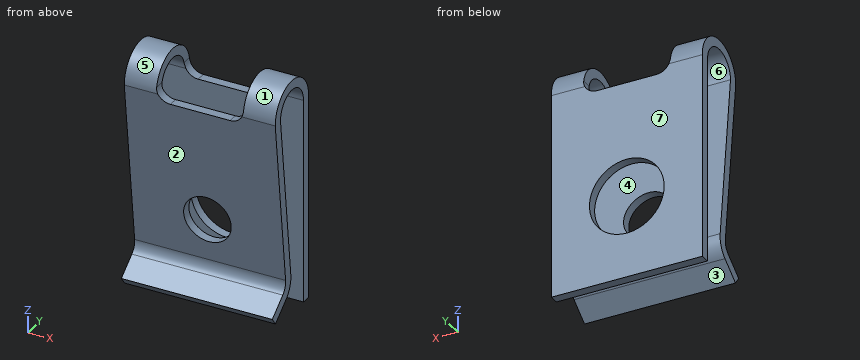
from build123d import *

# Parameters (mm, degrees)
F1_DEPTH = 5.56
F2_W     = 6.4
F2_H     = 3.95
F2_H_2   = 0.55
F2_R     = 1.75
F3_DEPTH = 4.901
F2_R_2   = 2.75
F4_DEPTH = 0.7
F5_R     = 1
F6_R     = 1.7


with BuildPart() as f1:
    # F0 (on Right) → F1 (new body, symmetric)
    with BuildSketch(Plane.YZ):
        with BuildLine():
            Line((1.55, -15), (2.25, -15))
            Line((2.25, -15), (2.25, 0))
            ThreePointArc((2.25, 0), (0, 2.25), (-2.25, 0))
            Line((-2.25, 0), (-0.790171, -12.749847))
            Line((-0.790171, -12.749847), (-2.65, -14.197634))
            Line((-2.65, -14.197634), (-2.22001, -14.75))
            Line((-2.22001, -14.75), (-0.05, -13.060752))
            Line((-0.05, -13.060752), (-1.549576, 0.036243))
            ThreePointArc((-1.549576, 0.036243), (0.018123, 1.549894), (1.55, 0))
            Line((1.55, 0), (1.55, -15))
        make_face()
    extrude(amount=F1_DEPTH, both=True)

    # F2 (on face) → F3 (cut, through all)
    with BuildSketch(Plane(origin=(0, 2.25, 0), x_dir=(-1, 0, 0), z_dir=(0, 1, 0))):
        with Locations((0, 1.975)):
            Rectangle(F2_W, F2_H)
        with Locations((0, -0.275)):
            Rectangle(F2_W, F2_H_2)
        with Locations((0, -9)):
            Circle(F2_R)
    extrude(amount=-F3_DEPTH, mode=Mode.SUBTRACT)

    # F2 (on face) → F4 (cut, through all)
    with BuildSketch(Plane(origin=(0, 2.25, 0), x_dir=(-1, 0, 0), z_dir=(0, 1, 0))):
        with Locations((0, -9)):
            Circle(F2_R_2)
        with Locations((0, -9)):
            Circle(F2_R, mode=Mode.SUBTRACT)
    extrude(amount=-F4_DEPTH, mode=Mode.SUBTRACT)

    # F5
    f5_edges = [f1.edges().sort_by_distance(p)[0] for p in [
        (-3.2, -1.83474, -0.55),
        (-3.2, 1.9, -0.55),
        (3.2, 1.9, -0.55),
        (3.2, -1.83474, -0.55),
        (0, -0.790171, -12.749847),
    ]]
    fillet(f5_edges, radius=F5_R)

    # F6
    f6_edges = [f1.edges().sort_by_distance(p)[0] for p in [
        (0, -0.05, -13.060752),
    ]]
    fillet(f6_edges, radius=F6_R)


solid = f1.part
Build history of the part. All positions in model axes, mm. Face numbers are marked on the shaded views. A direction names the side the tool comes from. Coordinates: 2 decimals unless noted, no trailing zeros. Write each loop counter-clockwise with the first axis right and the second up, starting at its lowest first coordinate (ties: lowest second). Pieces come first, ordered by that corner, then holes. Notation, with made-up numbers: (17, 89.25) -> (68, 89.25) arc R10 ccw to (68, 99.25) -> close; hole circle Ø3 at (13, 8.5). An arc over 180 degrees is marked (long way). Use CSV: the item, a comma, the result in double quotes. Start each with the question number.
Q1. Cut at A-A, the plane x = 0.5. List the corners of the cut face in (y, z).
Q2. Cut at C-C, the plane y = 1.3. List the corners of the cut face in (x, z), then the cut area to 3 significant figures.
Q3. Drill centre lines: probe 1 along Z at (x, y) = (0, 1.75); probe 2 along Y at (x, z) = (-5, -4.25); probe 3 along Y at (x, z) = (1, -1.5). Where is each one in solid material? Low to high.
Q4. 3-axis set-ups, long thin cutter, end or side, ignore diameter. For the marked faces 1, 2, 3 and 4: which of +Z, -Z, +X, -X, +Y, -Y reach the whole face in a straight line?
Q5. Pull direction Z, two halves, no side cores. Call the marked faces 5, 6 and 7: released by +Z, released by -Z, zero draft, split by the parting line, or undercut.
Q6. Flat gauge pins, fed straight in: pin 1 Ø4 at (x, z) = (0, -9) entering from +Y; pin 2 Ø4 at (x, z) = (1.5, -9.5) entering from -Y; pin 3 Ø0.6 at (x, y) = (0, 2) entering from +Z. Where does each tip first touch, or does it go through?
Q7. Cut at B-B, the plane z = -4.5. List the corners of the cut face in (x, y).
Q8. Cut at D-D, the plane z = -9. List the corners of the cut face in (x, y), then the cut area to 3 significant figures.
Checked values:
1,outline,"(-2.65, -14.2) -> (-2.22, -14.75) -> (-0.8, -13.65) arc R1.7 ccw to (-0.16, -12.11) -> (-0.32, -10.68) -> (-1.03, -10.68) -> (-0.85, -12.19) arc R1 cw to (-1.23, -13.09) -> close; (-2.19, -0.55) -> (-1.41, -7.32) -> (-0.71, -7.32) -> (-1.48, -0.55) -> close; (1.55, -15) -> (2.25, -15) -> (2.25, -11.7) -> (1.55, -11.7) -> close; (1.55, -6.3) -> (2.25, -6.3) -> (2.25, -0.55) -> (1.55, -0.55) -> close"
2,outline,"(-5.56, 0.84) -> (-3.2, 0.84) -> (-3.2, 1.84) -> (-5.56, 1.84) -> close; (3.2, 0.84) -> (5.56, 0.84) -> (5.56, 1.84) -> (3.2, 1.84) -> close"
2,area,"4.68 mm²"
3,probe 1,"z = -15 to -11.75, -6.25 to -0.55"
3,probe 2,"y = -1.76 to -1.06, 1.55 to 2.25"
3,probe 3,"y = -2.08 to -1.37, 1.55 to 2.25"
4,face 1,"+Z, +X, -X"
4,face 2,"+X, -X, -Y"
4,face 3,"-Z, +X, -X"
4,face 4,"+X, -X"
5,face 5,"released by +Z"
5,face 6,"undercut"
5,face 7,"zero draft"
6,pin 1,"stops at y = -0.29"
6,pin 2,"stops at y = -1.39"
6,pin 3,"stops at z = -0.55"
7,outline,"(-5.56, -1.73) -> (5.56, -1.73) -> (5.56, -1.03) -> (-5.56, -1.03) -> close; (-5.56, 1.55) -> (5.56, 1.55) -> (5.56, 2.25) -> (-5.56, 2.25) -> close"
8,outline,"(-5.56, -1.22) -> (-1.75, -1.22) -> (-1.75, -0.51) -> (-5.56, -0.51) -> close; (-5.56, 1.55) -> (-2.75, 1.55) -> (-2.75, 2.25) -> (-5.56, 2.25) -> close; (1.75, -1.22) -> (5.56, -1.22) -> (5.56, -0.51) -> (1.75, -0.51) -> close; (2.75, 1.55) -> (5.56, 1.55) -> (5.56, 2.25) -> (2.75, 2.25) -> close"
8,area,"9.30 mm²"
